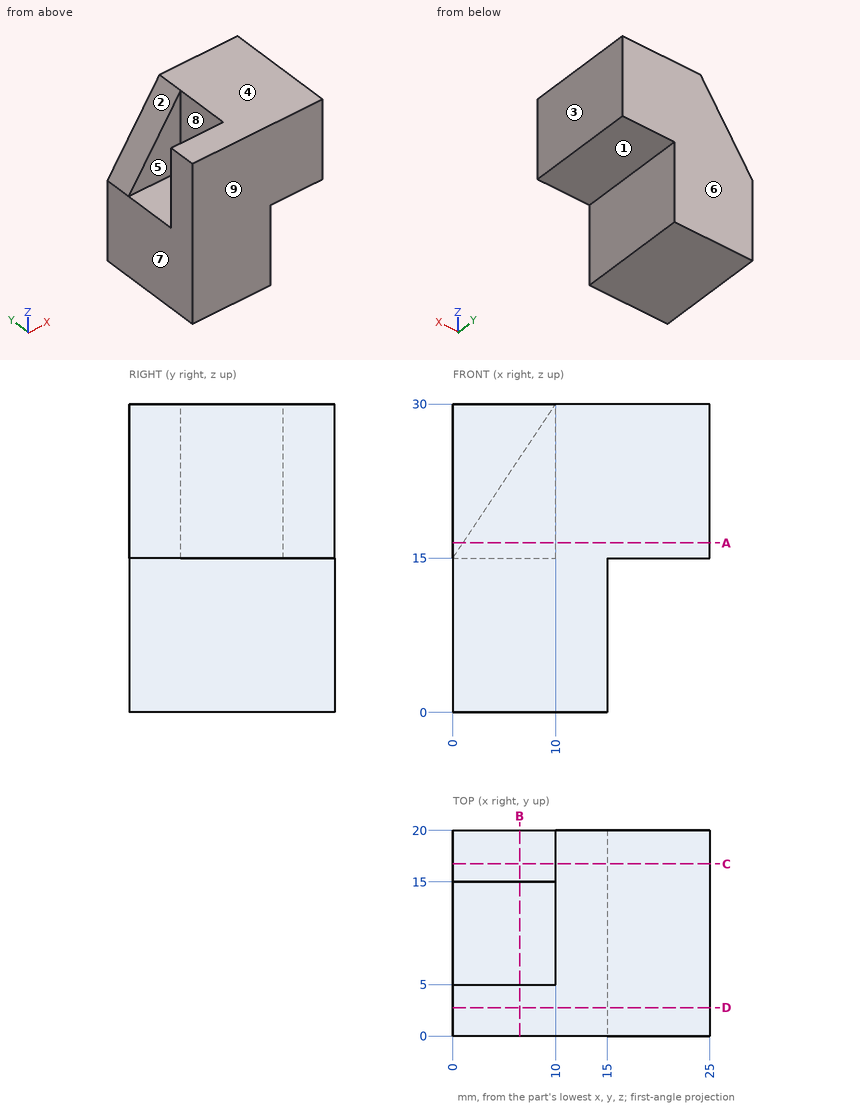
The figure shows three views and two pictorial views of one solid part (mm, origin at its lowest corner). Answer the questions. A direction names the side the tool comes from. Round coordinates to 2 decimals unless told otherwise and drop trailing zeros. Loops run counter-clockwise (first coordinate to the right, second up) from the corner with the lowest first, then second, coordinate; pieces in that order, holes last. Notation, with made-up numbers: (22, 54.25) - (64, 54.25) arc R14 cw to (64, 73.25) - close; hole circle Ø5 at (7, -34). An arc over 180 degrees is marked (long way). Use one line per item in the form item = value. Start each with the question number.
(1) Find section D-D on y = 2.75. Determine the outline of the cut face in (x, z).
(2) Find section B-B on x = 6.5. Determine the outline of the cut face in (y, z).
(3) Flat-ended cylindrical pins translate along their axes: P1, Ø2, axis at y = 3.5, z = 9.5, coming from the -X side; P2, Ø8, axis at x = 3.5, y = 10.5, coming from the +Z side; P3, Ø1, axis at x = 3, y = 15.5, coming from the +Z side; P4, Ø1, axis at y = 14, z = 23, coming from the -X side. Find the tip coordinate at first contact, or state that the pin passes through.
(4) Consider line 1 (Y direction, x = 3.75, z = 17); line 2 (Z direction, x = 16, y = 16.75); line 3 (X direction, y = 15.25, z = 1.75). Determine where each line is inside the solid, lowest interval first.
(5) Find section C-C on y = 16.75. Determine the outline of the cut face in (x, z), and give its area (3 significant figures).
(6) Find section A-A on z = 16.5. Determine the outline of the cut face in (x, y), and give its area (3 significant figures).
(7) Which of the six approach directions +Z, -Z, +X, -X, +Y, -Y give full straight-line access (tool end or side, diameter ignored) to the marked faces 1, 2, 3, 4 and 5?
(8) Determine the mould class of the marked faces 6, 7, 8 and 9 for opening direction Y: +Y half, -Y half, draft (parallel to the pull), parting line (faces both ways), or undercut.
Answer list:
q1.outline = (0, 0) - (15, 0) - (15, 15) - (25, 15) - (25, 30) - (0, 30) - close
q2.outline = (0, 0) - (20, 0) - (20, 24.75) - (15, 24.75) - (15, 15) - (5, 15) - (5, 30) - (0, 30) - close
q3.P1 = 0
q3.P2 = 15
q3.P3 = 20.25
q3.P4 = 10
q4.line_1 = 0 to 5, 15 to 20
q4.line_2 = 15 to 30
q4.line_3 = 0 to 15
q5.outline = (0, 0) - (15, 0) - (15, 15) - (25, 15) - (25, 30) - (10, 30) - (0, 15) - close
q5.area = 525 mm^2
q6.outline = (0, 0) - (25, 0) - (25, 20) - (1, 20) - (1, 15) - (10, 15) - (10, 5) - (0, 5) - close
q6.area = 395 mm^2
q7.face_1 = -Z, +X, +Y, -Y
q7.face_2 = +Z, -X, +Y
q7.face_3 = +Z, -Z, +X, +Y, -Y
q7.face_4 = +Z, +X, -X, +Y, -Y
q7.face_5 = +Z, -X
q8.face_6 = +Y half
q8.face_7 = draft
q8.face_8 = undercut
q8.face_9 = -Y half
